Build history of the part. All positions in model axes, mm. Give positions to 0.01 mm unless a question says otherwise; leave off trailing zeros. Order: outer loops, then holes, each group sorted by start corner. A loop starts at its lowest first (then second) coordinate and runs counter-clockwise, first axis right, second up. Notation, with made-up numbers: M 64,70.5 L 84,70.5 A16 cw 84,94.5 Z; hole C 12.5,8.25 d7. An arc over 180 degrees is marked long. One line per item, written item: value.
from build123d import *

# Parameters (mm, degrees)
SKETCH1_W           = 215
SKETCH1_H           = 227
SKETCH1_R           = 2.5
SKETCH1_W_2         = 45
SKETCH1_H_2         = 93
BOSS_EXTRUDE1_DEPTH = 7


with BuildPart() as part:
    # Sketch1 → Boss-Extrude1 (new body)
    with BuildSketch(Plane.XY):
        with Locations((0, 3.089375999)):
            Rectangle(SKETCH1_W, SKETCH1_H)
        with Locations((-13, -97.410624001)):
            Circle(SKETCH1_R, mode=Mode.SUBTRACT)
        with Locations((13, -97.410624001)):
            Circle(SKETCH1_R, mode=Mode.SUBTRACT)
        with Locations((0, 31.089375999)):
            Rectangle(SKETCH1_W_2, SKETCH1_H_2, mode=Mode.SUBTRACT)
    extrude(amount=BOSS_EXTRUDE1_DEPTH)


solid = part.part
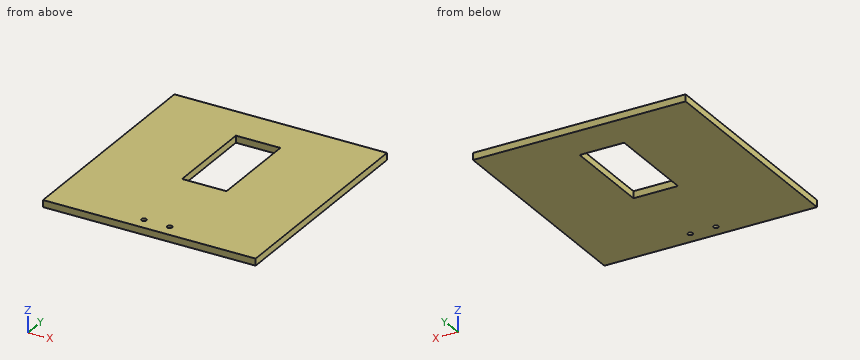
1) Pin check, flat tips, straight feed: pin 1 (1 mm diameter, centred on x = -55, y = 9, fed in from -Z); pin 2 (3 mm diameter, centred on x = 13, y = -97.41, fed in from +Z). Stop position of each tip, or through.
Check values:
pin 1: z = 0
pin 2: through
2) Saw through at A-A, the plane y = 67.5. Write the cut outline in (x, z), then the cut area to 3 significant figures.
Check values:
outline: M -107.5,0 L -22.5,0 L -22.5,7 L -107.5,7 Z; M 22.5,0 L 107.5,0 L 107.5,7 L 22.5,7 Z
area: 1,190 mm^2
3) Saw through at B-B, the plane z = 3.25. Write the cut outline in (x, y), then the cut area to 3 significant figures.
Check values:
outline: M -107.5,-110.41 L 107.5,-110.41 L 107.5,116.59 L -107.5,116.59 Z; hole M -22.5,-15.41 L 22.5,-15.41 L 22.5,77.59 L -22.5,77.59 Z; hole C -13,-97.41 d5; hole C 13,-97.41 d5
area: 44,600 mm^2
4) Drill centre lines: probe 1 along Y at (x, z) = (-13, 5); probe 2 along X at (y, z) = (41.5, 4.75); probe 3 along Y at (x, z) = (12.5, 5). Where is each one in solid material? Low to high. Write a range as from..to.
Check values:
probe 1: -110.41..-99.91, -94.91..-15.41, 77.59..116.59
probe 2: -107.5..-22.5, 22.5..107.5
probe 3: -110.41..-99.86, -94.96..-15.41, 77.59..116.59
